Can you work these out from the model? Positions are in its coordinate system, mm. Face numbers are marked on the shaded views. Give positions to 0.01 mm unless a question says otherwise; leave off trailing zeros. Order: outer loops, then holes, each group sorted by start corner. A loop starts at its lowest first (then second) coordinate and runs counter-clockwise, first axis right, second up.
Item 1: I want a section at A-A, the plane x = 0. Write out the boundary of the cut face in (y, z), then the cut area to 3 significant figures.
Item 2: I want a section at D-D, the plane x = 11. Write out the boundary of the cut face in (y, z), then the cut area to 3 significant figures.
Item 3: If we mould it in two halves opening along X, with no side actions, what happens to the marked faces 1, 2, 3 and 4? For each: +X half, -X half, draft (parallel to the pull), parting line (faces both ways), or undercut.
Item 4: If I drill on line 1 along Z through (x, y) = (0.5, 25.5); line 2 along Z through (x, y) = (20.5, 5.5); line 3 along X through (y, z) = (33.5, -42.75), over which ranges is the centre line in solid material (lowest first)?
Item 5: I want a section at B-B, the plane z = -43. Write out the boundary of the cut face in (x, y).
Item 6: I want a section at C-C, the plane y = 3. Write out the boundary of the cut face in (x, z), then the cut area to 3 significant figures.
Item 7: I'm going to push flat-ended pins straight in: pin 1 Ø1.5 at (y, z) = (9.5, -38.5) entering from +X; pin 2 Ø10 at (x, y) = (-18.5, 15.5) entering from -Z; pin 3 Ø2 at (y, z) = (19.5, -39.5) entering from -X. Where does each tip first touch, or does it pass through?
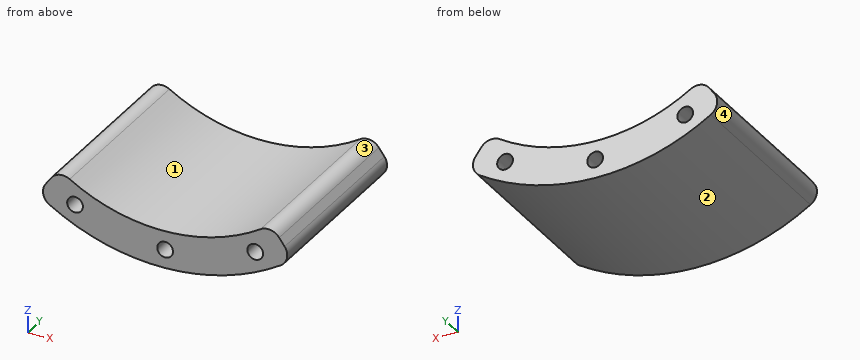
```python
from build123d import *

# Parameters (mm, degrees)
SKETCH_1_R      = 1.7
EXTRUDE_1_DEPTH = 40
FILLET_1_R      = 3


with BuildPart() as part:
    # 草图1 → 凸台-拉伸1 (new body)
    with BuildSketch(Plane(origin=(0, 0, 0), x_dir=(1, 0, 0), z_dir=(0, 1, 0))):
        with BuildLine():
            Line((-22.923624839, 31.551662781), (-27.625906858, 38.023798736))
            ThreePointArc((-27.625906858, 38.023798736), (0, 47), (27.625906858, 38.023798736))
            Line((27.625906858, 38.023798736), (22.923624839, 31.551662781))
            ThreePointArc((22.923624839, 31.551662781), (0, 39), (-22.923624839, 31.551662781))
        make_face()
        with Locations(Location((0, 43, 0), (0, 0, 270))):
            Circle(SKETCH_1_R, mode=Mode.SUBTRACT)
        with Locations(Location((19.451649922, 38.348837209, 0), (0, 0, 270))):
            Circle(SKETCH_1_R, mode=Mode.SUBTRACT)
        with Locations(Location((-19.451649922, 38.348837209, 0), (0, 0, 270))):
            Circle(SKETCH_1_R, mode=Mode.SUBTRACT)
    extrude(amount=EXTRUDE_1_DEPTH)

    # 圆角1
    fillet_1_edges = [part.edges().sort_by_distance(p)[0] for p in [
        (-22.923624839, 20, -31.551662781),
        (-27.625906858, 20, -38.023798736),
        (27.625906858, 20, -38.023798736),
        (22.923624839, 20, -31.551662781),
    ]]
    fillet(fillet_1_edges, radius=FILLET_1_R)


solid = part.part
```
Results list:
1. outline: (0, -47) - (40, -47) - (40, -44.7) - (0, -44.7) - close; (0, -41.3) - (40, -41.3) - (40, -39) - (0, -39) - close
1. area: 184 mm2
2. outline: (0, -45.69) - (40, -45.69) - (40, -37.42) - (0, -37.42) - close
2. area: 331 mm2
3. face 1: undercut
3. face 2: parting line
3. face 3: undercut
3. face 4: -X half
4. line 1: z = -47 to -44.62, -41.38 to -39
4. line 2: z = -42.29 to -39.69, -37.01 to -33.18
4. line 3: x = -19.53 to -1.68, 1.68 to 19.53
5. outline: (-18.97, 0) - (-1.7, 0) - (-1.7, 40) - (-18.97, 40) - close; (1.7, 0) - (18.97, 0) - (18.97, 40) - (1.7, 40) - close
6. outline: (-25.8, -35.51) arc R3 ccw to (-24.97, -39.82) arc R47 ccw to (24.97, -39.82) arc R3 ccw to (25.8, -35.51) - (24.62, -33.89) arc R3 ccw to (20.61, -33.11) arc R39 cw to (-20.61, -33.11) arc R3 ccw to (-24.62, -33.89) - close; hole circle Ø3.4 at (-19.45, -38.35); hole circle Ø3.4 at (0, -43); hole circle Ø3.4 at (19.45, -38.35)
6. area: 397 mm2
7. pin 1: stops at x = 26.34
7. pin 2: stops at z = -45.02
7. pin 3: stops at x = -26.11
